```python
from build123d import *

# Parameters (mm, degrees)
EXTRUDE_1_DEPTH     = 1.2
SKETCH_2_R          = 15.3
SKETCH_2_R_2        = 14.5
EXTRUDE_1_2_DEPTH   = 50
EXTRUDE_2_DEPTH     = 1.2
SKETCH_8_R          = 1.8
CUT_EXTRUDE_4_DEPTH = 2.2
SKETCH_2_2_R        = 14.5
CUT_EXTRUDE_1_DEPTH = 2.2
CUT_EXTRUDE_START   = -50
SKETCH_3_W          = 0.8
SKETCH_3_H          = 35
CUT_EXTRUDE_2_DEPTH = 50


with BuildPart() as part:
    # Sketch 1 → Extrude 1 (new body)
    with BuildSketch(Plane(origin=(0, 0, 0), x_dir=(1, 0, 0), z_dir=(0, 1, 0))):
        with BuildLine():
            Line((35, 0), (35, 15))
            Line((35, 15), (50, 15))
            Line((50, 15), (50, 0))
            ThreePointArc((50, 0), (7.5, -42.5), (-35, 0))
            ThreePointArc((-35, 0), (0, 35), (35, 0))
        make_face()
    extrude(amount=EXTRUDE_1_DEPTH)

    # Sketch 2 → Extrude 1 2 (add)
    with BuildSketch(Plane(origin=(0, 0, 0), x_dir=(1, 0, 0), z_dir=(0, 1, 0))):
        Circle(SKETCH_2_R)
        Circle(SKETCH_2_R_2, mode=Mode.SUBTRACT)
    extrude(amount=-EXTRUDE_1_2_DEPTH)

    # Sketch 7 → Extrude 2 (add)
    with BuildSketch(Plane(origin=(0, 0, 0), x_dir=(1, 0, 0), z_dir=(0, 1, 0))):
        with BuildLine():
            Line((36.331804249, 23), (58, 23))
            Line((58, 23), (58, 0))
            ThreePointArc((58, 0), (7.5, -50.5), (-43, 0))
            ThreePointArc((-43, 0), (-11.973562905, 41.299319502), (36.331804249, 23))
        make_face()
        with BuildLine():
            Line((35, 0), (35, 15))
            Line((35, 15), (50, 15))
            Line((50, 15), (50, 0))
            ThreePointArc((50, 0), (7.5, -42.5), (-35, 0))
            ThreePointArc((-35, 0), (0, 35), (35, 0))
        make_face(mode=Mode.SUBTRACT)
    extrude(amount=EXTRUDE_2_DEPTH)

    # Sketch 8 → Cut-Extrude 4 (cut, through all)
    with BuildSketch(Plane(origin=(0, 0, 0), x_dir=(1, 0, 0), z_dir=(0, 1, 0))):
        with Locations((34.058772732, 19)):
            Circle(SKETCH_8_R)
        with Locations((54, 19)):
            Circle(SKETCH_8_R)
        with Locations((54, 0)):
            Circle(SKETCH_8_R)
        with Locations((7.5, -46.5)):
            Circle(SKETCH_8_R)
        with Locations((-39, 0)):
            Circle(SKETCH_8_R)
        with Locations((0, 39)):
            Circle(SKETCH_8_R)
        with Locations((36.415922611, -36.415922611)):
            Circle(SKETCH_8_R)
        with Locations((-28.915922611, -28.915922611)):
            Circle(SKETCH_8_R)
        with Locations((-27.577164466, 27.577164466)):
            Circle(SKETCH_8_R)
        with Locations((27.577164466, 27.577164466)):
            Circle(SKETCH_8_R)
    extrude(amount=CUT_EXTRUDE_4_DEPTH, mode=Mode.SUBTRACT)

    # Sketch 2_2 → Cut-Extrude 1 (cut, through all)
    with BuildSketch(Plane(origin=(0, 0, 0), x_dir=(1, 0, 0), z_dir=(0, 1, 0))):
        Circle(SKETCH_2_2_R)
    extrude(amount=CUT_EXTRUDE_1_DEPTH, mode=Mode.SUBTRACT)

    # Sketch 3 → Cut-Extrude 2 (cut)
    with BuildSketch(Plane(origin=(0, 0, 0), x_dir=(1, 0, 0), z_dir=(0, 1, 0)).offset(CUT_EXTRUDE_START)):
        Rectangle(SKETCH_3_W, SKETCH_3_H)
    extrude(amount=CUT_EXTRUDE_2_DEPTH, mode=Mode.SUBTRACT)


solid = part.part
```
For this review, take the finished solid that the model builds, in its own axes (mm). A direction names the side the tool comes from. Coordinates: 2 decimals unless noted, no trailing zeros. Loops run counter-clockwise (first coordinate to the right, second up) from the corner with the lowest first, then second, coordinate; pieces in that order, holes last. Notation, with made-up numbers: (-9.5, -16) -> (30.5, -16) arc R30 ccw to (30.5, 13) -> close; hole circle Ø9 at (89, 26.5). An arc over 180 degrees is marked (long way). Return JSON: item names as keys, results as strings. Group by question number.
(1) Mouldability with a two-part tool opening along X and no side actions: class faces 1 (the cylindrical face through (8.61, 0.592, 50.488)), 2 (the flat face through (-15, -50, 0)), 3 (the cylindrical face through (25.78, 0.59, -27.66)) as pulls with the +X half, pulls with the -X half, needs draft (parallel to the pull), parting line crosses it, or undercut.
(2) To check wall thickness, follow L1, parallel to Z at x = 0, y = 0.45; L2, parallel to X at y = -26, z = 0; L3, parallel to X at y = 0.3, z = -19. State the ranges of each line that lie inside material, in increasing order.
(3) Tool access review of faces 4 (the cylindrical face through (15.296, -24.65, 0.331)), 5 (the cylindrical face through (-38.169, 0.592, 1.597)), 6 (the cylindrical face through (-15.296, -24.65, -0.331)): name each direction out of +Z, -Z, +X, -X, +Y, -Y from which nothing blocks a thin tool from reaching the whole face with its end or side.
(4) Consider section C-C, the plane z = -19. Give the boundary of the cut face in (x, y), plus the area to 3 significant figures.
(5) Consider section B-B, the plane x = -12.5. Give the boundary of the cut face in (y, z), plus the area to 3 significant figures.
(6) Consider section A-A, the plane y = -44. Give the boundary of the cut face in (x, z).
(7) Consider section D-D, the plane x = 7.5. Give the boundary of the cut face in (y, z), plus the area to 3 significant figures.
(8) For pin 1 Ø12 at (x, z) = (19.5, -18.5) entering from -Y; pin 2 Ø10 at (x, y) = (-8, -19.5) entering from +Z; pin 3 Ø4.5 at (x, z) = (54, -19) entering from +Y; pin 4 Ø3 at (y, z) = (-39, -11) entering from -X, all flat-tipped, find the tip position at first contact; note any pin that passes through.
Results below:
{
 "1": {"face 1": "parting line crosses it", "face 2": "needs draft", "face 3": "undercut"},
 "2": {"L1": "z = -43 to -40.8, -37.2 to -14.5, 14.5 to 49.94", "L2": "x = -15.3 to -14.5, 14.5 to 15.3", "L3": "x = -38.57 to 32.26, 35.86 to 52.2, 55.8 to 58"},
 "3": {"face 4": "+X, -Y", "face 5": "+Y, -Y", "face 6": "-X, -Y"},
 "4": {"outline": "(-38.57, 0) -> (32.26, 0) -> (32.26, 1.2) -> (-38.57, 1.2) -> close; (35.86, 0) -> (52.2, 0) -> (52.2, 1.2) -> (35.86, 1.2) -> close; (55.8, 0) -> (58, 0) -> (58, 1.2) -> (55.8, 1.2) -> close", "area": "107 mm2"},
 "5": {"outline": "(-50, -8.82) -> (0, -8.82) -> (0, -41.14) -> (1.2, -41.14) -> (1.2, -7.35) -> (-50, -7.35) -> close; (-50, 7.35) -> (1.2, 7.35) -> (1.2, 46.37) -> (0, 46.37) -> (0, 8.82) -> (-50, 8.82) -> close", "area": "235 mm2"},
 "6": {"outline": "(-0.4, -15.29) -> (-0.4, -14.49) arc R14.5 cw to (-0.4, 14.49) -> (-0.4, 15.29) arc R15.3 ccw to start; (0.4, -15.29) arc R15.3 ccw to (0.4, 15.29) -> (0.4, 14.49) arc R14.5 cw to (0.4, -14.49) -> close"},
 "7": {"outline": "(-50, -13.34) -> (0, -13.34) -> (0, -42.34) -> (1.2, -42.34) -> (1.2, -12.41) -> (-50, -12.41) -> close; (-50, 12.41) -> (1.2, 12.41) -> (1.2, 44.7) -> (0, 44.7) -> (0, 13.34) -> (-50, 13.34) -> close; (0, 48.3) -> (1.2, 48.3) -> (1.2, 50.5) -> (0, 50.5) -> close", "area": "170 mm2"},
 "8": {"pin 1": "stops at y = 0", "pin 2": "stops at z = 15", "pin 3": "stops at y = 1.2", "pin 4": "stops at x = -11.99"}
}
